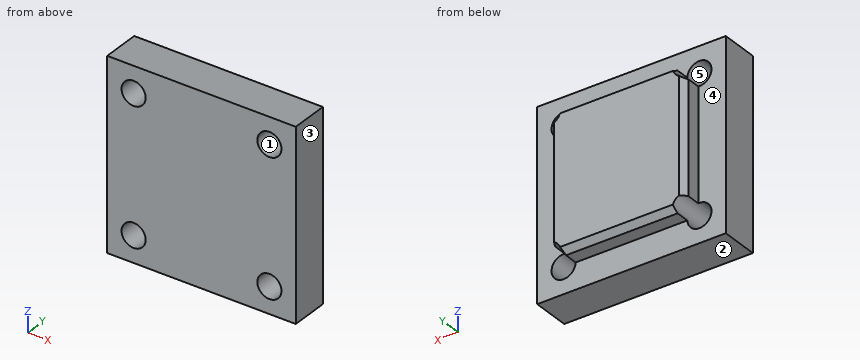
from build123d import *
from OCP.BRepFilletAPI import BRepFilletAPI_MakeChamfer

# Parameters (mm, degrees)
SKETCH1_W               = 25
SKETCH1_H               = 25
BOSS_EXTRUDE1_DEPTH     = 5
SKETCH4_R               = 4.15
CUT_EXTRUDE2_DEPTH      = 19.371173071
SKETCH9_W               = 17.7
SKETCH9_H               = 18.092678694
BOSS_EXTRUDE3_DEPTH     = 2.8
CUT_EXTRUDE4_DEPTH      = 19.371173071
CUT_EXTRUDE4_DEPTH_BACK = 19.371173071
SKETCH6_R               = 1.6
CHAMFER1_SIZE           = 1
CHAMFER1_SIZE2          = 0.577350269
SKETCH10_R              = 4.15
BOSS_EXTRUDE4_DEPTH     = 5


with BuildPart() as part:
    # Sketch1 → Boss-Extrude1 (new body)
    with BuildSketch(Plane(origin=(0, 0, 0), x_dir=(1, 0, 0), z_dir=(0, 1, 0))):
        Rectangle(SKETCH1_W, SKETCH1_H)
    extrude(amount=BOSS_EXTRUDE1_DEPTH)

    # Sketch4 → Cut-Extrude2 (cut, through all)
    with BuildSketch(Plane(origin=(0, 5, 0), x_dir=(1, 0, 0), z_dir=(0, 1, 0))):
        with Locations(Location((0, 0, 0), (0, 0, 270))):
            Circle(SKETCH4_R)
    extrude(amount=-CUT_EXTRUDE2_DEPTH, mode=Mode.SUBTRACT)

    # Sketch9 → Boss-Extrude3 (add)
    with BuildSketch(Plane(origin=(0, 5, 0), x_dir=(1, 0, 0), z_dir=(0, 1, 0))):
        Rectangle(SKETCH9_W, SKETCH9_H)
    extrude(amount=BOSS_EXTRUDE3_DEPTH)

    # Sketch6 → Cut-Extrude4 (cut, two sides: drawn at the far end of the back side and taken through both)
    with BuildSketch(Plane(origin=(0, 5, 0), x_dir=(1, 0, 0), z_dir=(0, 1, 0)).offset(-CUT_EXTRUDE4_DEPTH_BACK)):
        with Locations(Location((9, -9, 0), (0, 0, 270))):
            Circle(SKETCH6_R)
        with Locations(Location((-9, -9, 0), (0, 0, 270))):
            Circle(SKETCH6_R)
        with Locations(Location((-9, 9, 0), (0, 0, 270))):
            Circle(SKETCH6_R)
        with Locations(Location((9, 9, 0), (0, 0, 270))):
            Circle(SKETCH6_R)
    extrude(amount=CUT_EXTRUDE4_DEPTH + CUT_EXTRUDE4_DEPTH_BACK, mode=Mode.SUBTRACT)

    # Chamfer1: one chamfer whose edges measure the first distance from different faces: ONE call of the kernel's chamfer builder (chamfer() names one face for all edges)
    chamfer1_edges_1 = [part.edges().sort_by_distance(p)[0] for p in [
        (8.85, 7.8, 0),
    ]]
    chamfer1_side_1 = [part.faces().sort_by_distance(p)[0] for p in [
        (8.85, 6.4, 0),
    ]]
    chamfer1_edges_2 = [part.edges().sort_by_distance(p)[0] for p in [
        (0, 7.8, 9.046339347),
    ]]
    chamfer1_side_2 = [part.faces().sort_by_distance(p)[0] for p in [
        (0, 6.4, 9.046339347),
    ]]
    chamfer1_edges_3 = [part.edges().sort_by_distance(p)[0] for p in [
        (0, 7.8, -9.046339347),
    ]]
    chamfer1_side_3 = [part.faces().sort_by_distance(p)[0] for p in [
        (0, 6.4, -9.046339347),
    ]]
    chamfer1_edges_4 = [part.edges().sort_by_distance(p)[0] for p in [
        (-8.85, 7.8, 0),
    ]]
    chamfer1_side_4 = [part.faces().sort_by_distance(p)[0] for p in [
        (-8.85, 6.4, 0),
    ]]
    chamfer1 = BRepFilletAPI_MakeChamfer(part.part.solid().wrapped)
    for e in chamfer1_edges_1:
        chamfer1.Add(CHAMFER1_SIZE, CHAMFER1_SIZE2, e.wrapped, chamfer1_side_1[0].wrapped)  # the first distance lies on this face
    for e in chamfer1_edges_2:
        chamfer1.Add(CHAMFER1_SIZE, CHAMFER1_SIZE2, e.wrapped, chamfer1_side_2[0].wrapped)  # the first distance lies on this face
    for e in chamfer1_edges_3:
        chamfer1.Add(CHAMFER1_SIZE, CHAMFER1_SIZE2, e.wrapped, chamfer1_side_3[0].wrapped)  # the first distance lies on this face
    for e in chamfer1_edges_4:
        chamfer1.Add(CHAMFER1_SIZE, CHAMFER1_SIZE2, e.wrapped, chamfer1_side_4[0].wrapped)  # the first distance lies on this face
    add(Compound.cast(chamfer1.Shape()), mode=Mode.REPLACE)

    # Sketch10 → Boss-Extrude4 (add)
    with BuildSketch(Plane.XZ.offset(-5)):
        Circle(SKETCH10_R)
    extrude(amount=BOSS_EXTRUDE4_DEPTH)


solid = part.part
Can you work these out from the model? Positions are in its coordinate system, mm. Face numbers are marked on the shaded views. A direction names the side the tool comes from. Round coordinates to 2 decimals unless told otherwise and drop trailing zeros. Write each loop counter-clockwise with the first axis right and the second up, starting at its lowest first coordinate (ties: lowest second). Pieces come first, ordered by that corner, then holes. Notation, with made-up numbers: M -20.5,-17 L -15.5,-17 A31 cw -15.5,13 Z; hole C -39,28 d11. An arc over 180 degrees is marked long. Use a Markdown table: item, result.
Item 1: We'd pull the mould along Z, two halves only. Please class the marked faces 1, 2 and 3: released by +Z, released by -Z, zero draft, split by the parting line, or undercut.
Found:
| item | result |
|---|---|
| face 1 | undercut |
| face 2 | released by -Z |
| face 3 | zero draft |
Item 2: For pin 1 Ø1.4 at (y, z) = (5.5, 1.5) entering from +X; pin 2 Ø0.9 at (x, y) = (1, 6) entering from -Z; pin 3 Ø0.5 at (y, z) = (6, 1) entering from -X, each with a flat end and sliding along its axis, tell me the tip position at first contact or that it passes through.
Found:
| item | result |
|---|---|
| pin 1 | stops at x = 12.5 |
| pin 2 | stops at z = -9.05 |
| pin 3 | stops at x = -8.85 |
Item 3: If I drill on line 1 along Z through (x, y) = (9, 3.5); line 2 along X through (y, z) = (4.5, -9.5), over which ranges is the centre line in solid material (lowest first)? Write a range as [from, to].
Found:
| item | result |
|---|---|
| line 1 | z = [-12.5, -10.6], [-7.4, 7.4], [10.6, 12.5] |
| line 2 | x = [-12.5, -10.52], [-7.48, 7.48], [10.52, 12.5] |
Item 4: I want a section at A-A (y = 1). List the corners of the cut face in (x, z) for me, and give its area (3 significant figures).
Found:
| item | result |
|---|---|
| outline | M -12.5,-12.5 L 12.5,-12.5 L 12.5,12.5 L -12.5,12.5 Z; hole C -9,-9 d3.2; hole C -9,9 d3.2; hole C 9,-9 d3.2; hole C 9,9 d3.2 |
| area | 593 mm2 |
Item 5: I want a section at B-B (x = 10.25). List the corners of the cut face in (y, z) for me, and give its area (3 significant figures).
Found:
| item | result |
|---|---|
| outline | M 0,-12.5 L 5,-12.5 L 5,-10 L 0,-10 Z; M 0,-8 L 5,-8 L 5,8 L 0,8 Z; M 0,10 L 5,10 L 5,12.5 L 0,12.5 Z |
| area | 105 mm2 |
Item 6: Which directions (+Z, -Z, +X, -X, +Y, -Y) give clear straight access to the entire face, cutting with the end or side of a thin tool? Please do the marked faces 4 and 5.
Found:
| item | result |
|---|---|
| face 4 | +Y |
| face 5 | +Y, -Y |
Item 7: I want a section at D-D (x = -1). List the corners of the cut face in (y, z) for me, and give its area (3 significant figures).
Found:
| item | result |
|---|---|
| outline | M 0,-12.5 L 5,-12.5 L 5,-9.05 L 6.8,-9.05 L 7.8,-8.47 L 7.8,8.47 L 6.8,9.05 L 5,9.05 L 5,12.5 L 0,12.5 Z |
| area | 175 mm2 |
Item 8: I want a section at C-C (z = 4.25). List the corners of the cut face in (x, y) for me.
Found:
| item | result |
|---|---|
| outline | M -12.5,0 L 12.5,0 L 12.5,5 L 8.85,5 L 8.85,6.8 L 8.27,7.8 L -8.27,7.8 L -8.85,6.8 L -8.85,5 L -12.5,5 Z |
